Answer from the drawing. Dimensions are ordinates in mm from the lowest x, y and z of the part. Give positions to 0.01 mm unless a question says otherwise; leave off trailing zeros. Order: outer loops, then holes, each group sorted by start corner. A loop starts at its lowest first (then second) coordinate and runs counter-clockwise, first axis right, second up. Notation, with made-up numbers: (61.25, 55) - (99.25, 55) arc R38 cw to (99.25, 93) - close; hole circle Ø5 at (13, -17.5). An arc over 180 degrees is marked (long way). Use a Markdown table: item, result. Add a question column.
1) Find section A-A, the plane x = 12.5. Determine the outline of the cut face in (y, z), plus the area to 3 significant figures.
2) Find section C-C, the plane y = 0.95. State how many separate pieces and enclosed holes the cut face has, plus the area to 3 significant figures.
3) Flat-ended cylindrical pins translate along their axes: pin 1 (4 mm diameter, centred on x = 3, z = 26.5, fed in from +Y); pin 2 (2.5 mm diameter, centred on x = 31, z = 26.5, fed in from +Y); pin 3 (0.5 mm diameter, centred on x = 2, y = 0.5, fed in from -Z). Find the tip coordinate at first contact, or state that the pin passes through.
4) Straight lines are drawn through the part: line 1 (X direction, y = 0.65, z = 26.5); line 2 (X direction, y = 1.45, z = 13.75); line 3 (X direction, y = 1.15, z = 4.5). For each, find the intervals that lie inside material, in ascending order.
5) Find section B-B, the plane z = 12.25. Determine the outline of the cut face in (x, y).
6) Find section D-D, the plane x = 31. Determine the outline of the cut face in (y, z), plus the area to 3 significant figures.
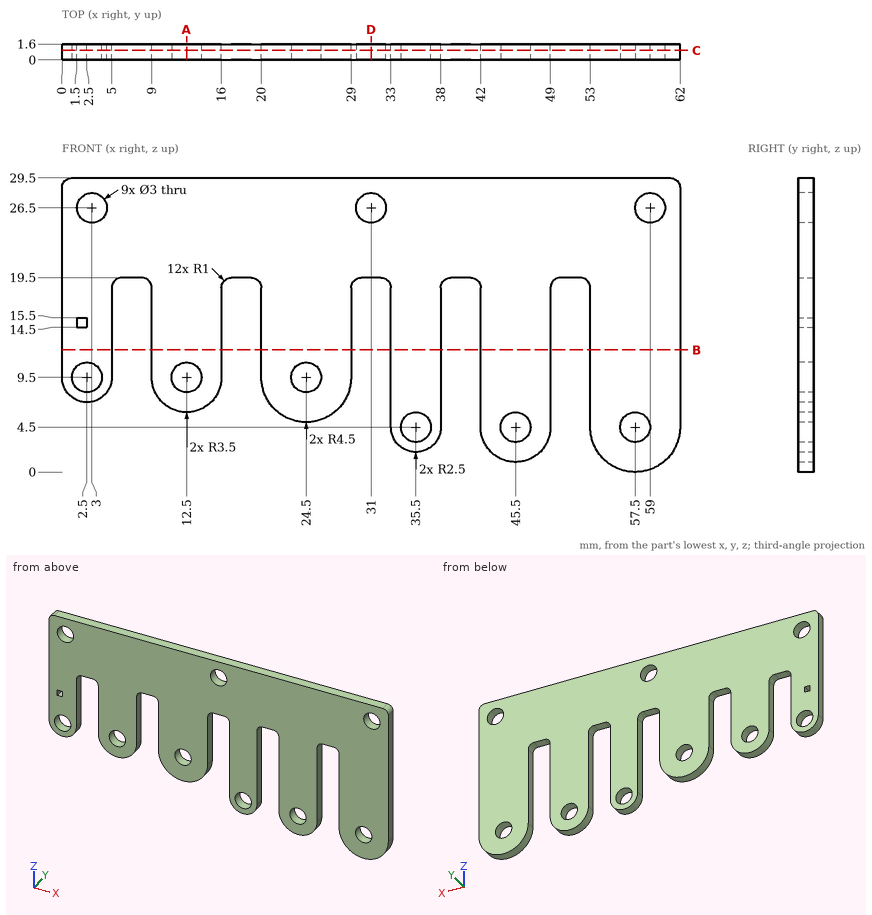
The answers:
| question | item | result |
|---|---|---|
| 1 | outline | (0, 6) - (1.6, 6) - (1.6, 8) - (0, 8) - close; (0, 11) - (1.6, 11) - (1.6, 29.5) - (0, 29.5) - close |
| 1 | area | 32.8 mm2 |
| 2 | separate pieces | 1 |
| 2 | enclosed holes | 10 |
| 2 | area | 1,200 mm2 |
| 3 | pin 1 | y = 1.6 |
| 3 | pin 2 | through |
| 3 | pin 3 | z = 7.01 |
| 4 | line 1 | 0 to 1.5, 4.5 to 29.5, 32.5 to 57.5, 60.5 to 62 |
| 4 | line 2 | 0 to 5, 9 to 16, 20 to 29, 33 to 38, 42 to 49, 53 to 62 |
| 4 | line 3 | 33 to 34, 37 to 38, 42 to 44, 47 to 49, 53 to 56, 59 to 62 |
| 5 | outline | (0, 0) - (5, 0) - (5, 1.6) - (0, 1.6) - close; (9, 0) - (16, 0) - (16, 1.6) - (9, 1.6) - close; (20, 0) - (29, 0) - (29, 1.6) - (20, 1.6) - close; (33, 0) - (38, 0) - (38, 1.6) - (33, 1.6) - close; (42, 0) - (49, 0) - (49, 1.6) - (42, 1.6) - close; (53, 0) - (62, 0) - (62, 1.6) - (53, 1.6) - close |
| 6 | outline | (0, 19.5) - (1.6, 19.5) - (1.6, 25) - (0, 25) - close; (0, 28) - (1.6, 28) - (1.6, 29.5) - (0, 29.5) - close |
| 6 | area | 11.2 mm2 |
